```python
from build123d import *

# Parameters (mm, degrees)
SKETCH1_R           = 235
BOSS_EXTRUDE1_DEPTH = 350
SKETCH3_R           = 50
CUT_EXTRUDE1_DEPTH  = 250
FILLET1_R           = 100


with BuildPart() as part:
    # Sketch1 → Boss-Extrude1 (new body)
    with BuildSketch(Plane(origin=(0, 0, 0), x_dir=(1, 0, 0), z_dir=(0, 1, 0))):
        Circle(SKETCH1_R)
    extrude(amount=BOSS_EXTRUDE1_DEPTH)

    # Sketch3 → Cut-Extrude1 (cut)
    with BuildSketch(Plane(origin=(0, 350, 0), x_dir=(1, 0, 0), z_dir=(0, 1, 0))):
        Circle(SKETCH3_R)
    extrude(amount=-CUT_EXTRUDE1_DEPTH, mode=Mode.SUBTRACT)

    # Fillet1
    fillet1_edges = [part.edges().sort_by_distance(p)[0] for p in [
        (-235, 350, 0),
    ]]
    fillet(fillet1_edges, radius=FILLET1_R)


solid = part.part
```
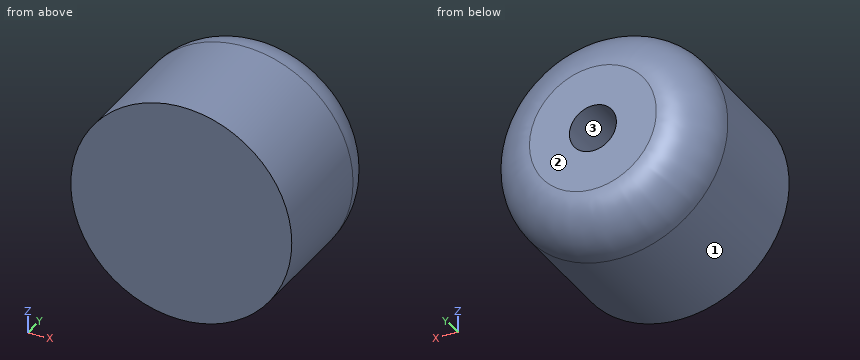
The model under review builds one solid part; all positions refer to its coordinate system, in mm. Face numbers are marked on the shaded views. Round coordinates to 2 decimals unless told otherwise and drop trailing zeros. Order: outer loops, then holes, each group sorted by start corner. A loop starts at its lowest first (then second) coordinate and runs counter-clockwise, first axis right, second up. Notation, with made-up numbers: (87.5, 16.5) -> (142.5, 16.5) arc R4 cw to (142.5, 23.5) -> close; hole circle Ø1 at (32.5, 86). An arc over 180 degrees is marked (long way). One line per item, written item: value. Start each with the question number.
Q1. Mouldability with a two-part tool opening along Z and no side actions: class the marked faces 1, 2 and 3 as released by +Z, released by -Z, zero draft, split by the parting line, or undercut.
Q2. Wall thickness on line 1 (Z direction, x = 0, y = 174); line 2 (X direction, y = 285.5, z = 0): over which ranges is each line inside the solid? List them lowest first.
Q3. Clearance check with flat-ended pins moving along their axes: pin 1 Ø3 at (y, z) = (59.5, -151.5) entering from -X; pin 2 Ø8 at (y, z) = (85.5, 112) entering from +X; pin 3 Ø2 at (y, z) = (85.5, -158.5) entering from +X. State where each tip first meets the part, or that it passes through.
Q4. Take a section at C-C (y = 166.5). Write out the cut boundary in (x, z).
Q5. Take a section at A-A (x = 0). Write out the cut boundary in (y, z).
Q6. Take a section at B-B (z = 0). Write out the cut boundary in (x, y).
Q7. Take a section at D-D (y = 45). Write out the cut boundary in (x, z), and give its area (3 significant figures).
Reported:
1. face 1: split by the parting line
1. face 2: zero draft
1. face 3: undercut
2. line 1: z = -235 to -50, 50 to 235
2. line 2: x = -228.49 to -50, 50 to 228.49
3. pin 1: stops at x = -180.9
3. pin 2: stops at x = 208.71
3. pin 3: stops at x = 174.41
4. outline: circle Ø470 at (0, 0); hole circle Ø100 at (0, 0)
5. outline: (0, -235) -> (250, -235) arc R100 ccw to (350, -135) -> (350, -50) -> (100, -50) -> (100, 50) -> (350, 50) -> (350, 135) arc R100 ccw to (250, 235) -> (0, 235) -> close
6. outline: (-235, 0) -> (235, 0) -> (235, 250) arc R100 ccw to (135, 350) -> (50, 350) -> (50, 100) -> (-50, 100) -> (-50, 350) -> (-135, 350) arc R100 ccw to (-235, 250) -> close
7. outline: circle Ø470 at (0, 0)
7. area: 173,000 mm2
